The model under review builds one solid part; all positions refer to its coordinate system, in mm. A direction names the side the tool comes from. Give positions to 0.01 mm unless a question says otherwise; leave off trailing zeros. Order: outer loops, then holes, each group sorted by start corner. A loop starts at its lowest first (then second) coordinate and runs counter-clockwise, first axis right, second up. Notation, with made-up numbers: (-29, -29) - (-18, -29) arc R7 cw to (-18, -20) - close; hole circle Ø2 at (-30.5, 30). An arc over 180 degrees is marked (long way). Put each result on its own line as item: value.
```python
from build123d import *

# Parameters (mm, degrees)
F0_R     = 32.5
F1_DEPTH = 2
F2_R     = 31.3
F3_DEPTH = 1
F4_R     = 22.5
F5_DEPTH = 1


with BuildPart() as f1:
    # F0 (on Top) → F1 (new body)
    with BuildSketch(Plane.XY):
        Circle(F0_R)
    extrude(amount=F1_DEPTH)

    # F2 (on face) → F3 (cut)
    with BuildSketch(Plane.XY.offset(2)):
        Circle(F2_R)
    extrude(amount=-F3_DEPTH, mode=Mode.SUBTRACT)

    # F4 (on face) → F5 (join)
    with BuildSketch(Plane.XY.offset(1)):
        Circle(F4_R)
        with BuildLine():
            ThreePointArc((0, -21.3), (-8.482899, 0), (0, 21.3))
            ThreePointArc((0, 21.3), (21.3, 0), (0, -21.3))
        make_face(mode=Mode.SUBTRACT)
    extrude(amount=F5_DEPTH)


solid = f1.part
```
(1) The part is to be moulded in two halves that separate along Y. For faces 3 (the flat face through (-10, -2, 2)), 4 (the cylindrical face through (31, 9.76, 0.99)), 5 (the flat face through (6, 0, 1)), say which applies: pulls with the +Y half, pulls with the -Y half, needs draft (parallel to the pull), parting line crosses it, or undercut.
The answers:
face 3: needs draft
face 4: parting line crosses it
face 5: undercut
(2) Take a section at A-A, the plane y = 0. Write out the cut boundary in (x, z).
The answers:
outline: (-32.5, 0) - (32.5, 0) - (32.5, 2) - (31.3, 2) - (31.3, 1) - (22.5, 1) - (22.5, 2) - (21.3, 2) - (21.3, 1) - (-8.48, 1) - (-8.48, 2) - (-22.5, 2) - (-22.5, 1) - (-31.3, 1) - (-31.3, 2) - (-32.5, 2) - close
(3) Take a section at B-B, the plane x = -13. Write out the cut boundary in (y, z), then the cut area to 3 significant figures.
The answers:
outline: (-29.79, 0) - (29.79, 0) - (29.79, 2) - (28.47, 2) - (28.47, 1) - (18.36, 1) - (18.36, 2) - (-18.36, 2) - (-18.36, 1) - (-28.47, 1) - (-28.47, 2) - (-29.79, 2) - close
area: 98.9 mm^2
(4) For faces 1 (the flat face through (-17, 27, 2)), 2 (the cylindrical face through (21.295, 0.468, 1.493)), list the 3-axis set-ups (+Z, -Z, +X, -X, +Y, -Y) from which the entire face can be reached by the end or side of a thin tool; tool diameter is ignored.
The answers:
face 1: +Z, +X, -X, +Y, -Y
face 2: +Z
(5) Wall thickness on L1, parallel to Y at x = 0, z = 1.6; L2, parallel to X at y = -11, z = 1.95; L3, parallel to Y at x = -0.5, z = 1.25: over which ranges is each line inside the solid? List them lowest first.
The answers:
L1: -32.5 to -31.3, -22.5 to -21.3, 21.3 to 22.5, 31.3 to 32.5
L2: -30.58 to -29.3, -19.63 to -6.46, 18.24 to 19.63, 29.3 to 30.58
L3: -32.5 to -31.3, -22.49 to -20.76, 20.76 to 22.49, 31.3 to 32.5
(6) Take a section at C-C, the plane z = 0.45. Write out the cut boundary in (x, y).
The answers:
outline: circle Ø65 at (0, 0)
(7) Clearance check with flat-ended pins moving along their axes: pin 1 Ø1 at (y, z) = (5.5, 0.5) entering from -X; pin 2 Ø9 at (x, y) = (8, -2.5) entering from +Z. State where each tip first meets the part, or that it passes through.
The answers:
pin 1: x = -32.11
pin 2: z = 1
(8) Take a section at D-D, the plane x = 27. Write out the cut boundary in (y, z).
The answers:
outline: (-18.09, 0) - (18.09, 0) - (18.09, 2) - (15.83, 2) - (15.83, 1) - (-15.83, 1) - (-15.83, 2) - (-18.09, 2) - close
